For this review, take the finished solid that the model builds, in its own axes (mm). A direction names the side the tool comes from. Give positions to 0.01 mm unless a question says otherwise; leave off trailing zeros. Write each loop counter-clockwise with the first axis right and the second up, starting at its lowest first coordinate (ties: lowest second). Pieces come first, ordered by that corner, then holes. Notation, with made-up numbers: (17.5, 35) -> (74.5, 35) arc R15 cw to (74.5, 63) -> close; hole circle Ø5 at (-1, -23). An arc over 180 degrees is marked (long way). Write item = value, one per line.
```python
from build123d import *

# Parameters (mm, degrees)
BOSS_EXTRU_1_DEPTH      = 50
ESQUISSE3_R             = 20
ENL_V_MAT_EXTRU_1_DEPTH = 10
CONG_1_R                = 15
CONG_2_R                = 5
CONG_4_R                = 10
CONG_5_R                = 10


with BuildPart() as part:
    # Esquisse2 → Boss.-Extru.1 (new body)
    with BuildSketch(Plane.XY):
        Polygon((-35, 90), (-85, 90), (-85, 50), (0, 50), (0, 0), (25, 0), (25, 60), (-75, 60), (-75, 80), (-35, 80), align=None)
    extrude(amount=BOSS_EXTRU_1_DEPTH)

    # Esquisse3 → Enlèv. mat.-Extru.1 (cut)
    with BuildSketch(Plane(origin=(0, 90, 0), x_dir=(1, 0, 0), z_dir=(0, 1, 0))):
        with Locations((-35, -25)):
            Circle(ESQUISSE3_R)
    extrude(amount=-ENL_V_MAT_EXTRU_1_DEPTH, mode=Mode.SUBTRACT)

    # Congé1
    cong_1_edges = [part.edges().sort_by_distance(p)[0] for p in [
        (0, 50, 25),
        (-75, 60, 25),
    ]]
    fillet(cong_1_edges, radius=CONG_1_R)

    # Congé2
    cong_2_edges = [part.edges().sort_by_distance(p)[0] for p in [
        (-75, 80, 25),
    ]]
    fillet(cong_2_edges, radius=CONG_2_R - 0.0001)  # a hair under: the kernel refuses the full size

    # Congé4
    cong_4_edges = [part.edges().sort_by_distance(p)[0] for p in [
        (-85, 50, 25),
        (-85, 90, 25),
    ]]
    fillet(cong_4_edges, radius=CONG_4_R)

    # Congé5
    cong_5_edges = [part.edges().sort_by_distance(p)[0] for p in [
        (-35, 90, 2.5),
        (-35, 90, 47.5),
    ]]
    fillet(cong_5_edges, radius=CONG_5_R - 0.0001)  # a hair under: the kernel refuses the full size


solid = part.part
```
(1) Take a section at C-C (y = 52). Write out the cut boundary in (x, z), plus the area to 3 significant figures.
Answers below:
outline = (-81, 0) -> (25, 0) -> (25, 50) -> (-81, 50) -> close
area = 5,300 mm^2
(2) The part is to be moulded in two halves that separate along Z. For faces 4 (the face through (0, 18, 25)), 5 (the face through (-22, 55, 0)), 6 (the face through (-55, 85, 25)), say which applies: released by +Z, released by -Z, zero draft, split by the parting line, or undercut.
Answers below:
face_4 = zero draft
face_5 = released by -Z
face_6 = undercut
(3) For pin 1 (15 mm diameter, centred on x = -41, z = 25.5, fed in from -Y); pin 2 (25 mm diameter, centred on x = -21.5, z = 30.5, fed in from +Y); pin 3 (5 mm diameter, centred on y = 51, z = 39.5, fed in from -X), all flat-tipped, find the tip position at first contact; note any pin that passes through.
Answers below:
pin_1 = 50
pin_2 = 60
pin_3 = -82.6
(4) Tool access review of faces 1 (the face through (-45, 50, 25)), 2 (the face through (-38.01, 87.15, 47.07)), 3 (the face through (-17, 60, 25)): name each direction out of +Z, -Z, +X, -X, +Y, -Y from which nothing blocks a thin tool from reaching the whole face with its end or side.
Answers below:
face_1 = +Z, -Z, -X, -Y
face_2 = +Z, -Z, +X, +Y
face_3 = +Z, -Z, +X
(5) Take a section at B-B (x = -41). Write out the cut boundary in (y, z), plus the area to 3 significant figures.
Answers below:
outline = (50, 0) -> (60, 0) -> (60, 50) -> (50, 50) -> close; (80, 0) -> (89.17, 0) -> (89.17, 5.92) -> (80, 5.92) -> close; (80, 44.08) -> (89.17, 44.08) -> (89.17, 50) -> (80, 50) -> close
area = 609 mm^2
(6) To check wall thickness, follow probe 1 along Y at (x, z) = (-57, 18); probe 2 along X at (y, z) = (21, 6); probe 3 along Y at (x, z) = (-48, 12). State the ranges of each line that lie inside material, in increasing order.
Answers below:
probe_1 = 50 to 60, 80 to 90
probe_2 = 0 to 25
probe_3 = 50 to 60
